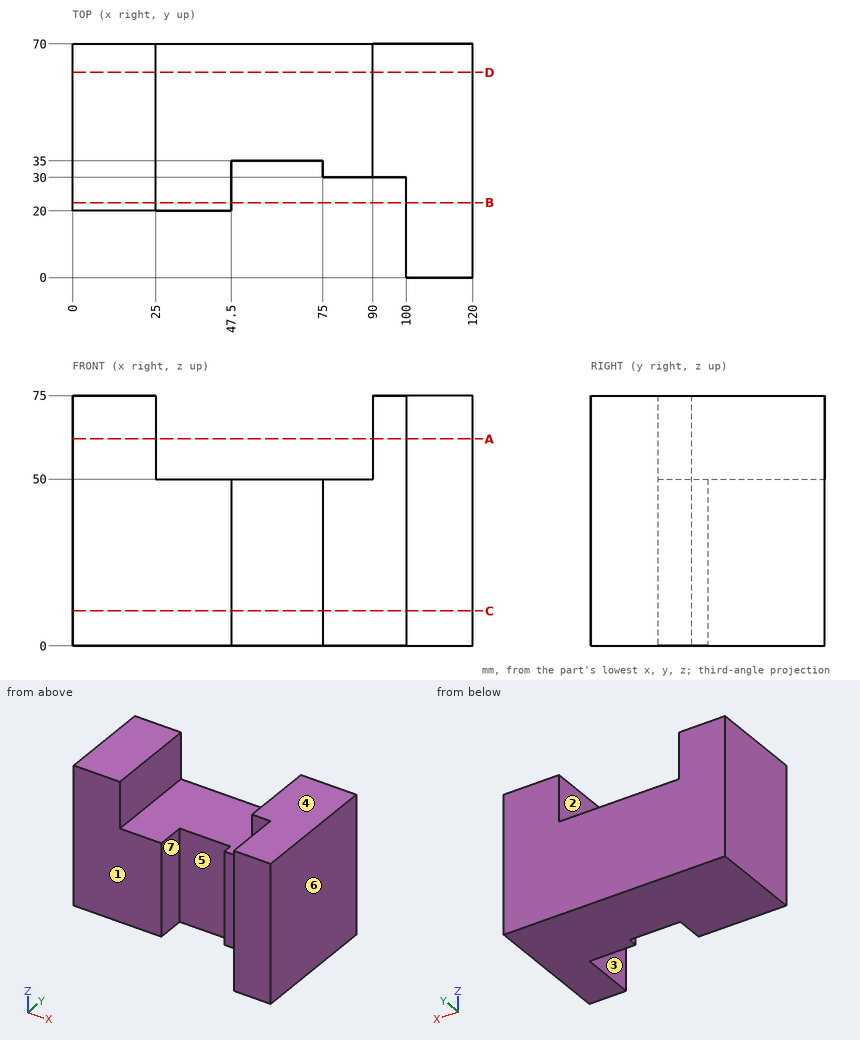
Drawing for the job (mm, zero at the part's lowest x, y, z). A direction names the side the tool comes from. Give positions to 0.01 mm unless a question says otherwise; leave off trailing zeros. Order: outer loops, then holes, each group sorted by start corner. A loop starts at its lowest first (then second) coordinate and runs counter-clockwise, first axis right, second up. Notation, with made-up numbers: (40.25, 8) - (66.25, 8) arc R18 cw to (66.25, 17) - close; hole circle Ø4 at (88.5, 87). An arc over 180 degrees is marked (long way). Use one line per item in the form item = value.
Item 1: Slice it at D-D on y = 61.5. Give the cut face in (x, z).
Solution:
outline = (0, 0) - (120, 0) - (120, 75) - (90, 75) - (90, 50) - (25, 50) - (25, 75) - (0, 75) - close
Item 2: Two-plate mould, pull along X, no slides. Class the marked faces 4, 5, 6 and 7: released by +X, released by -X, zero draft, split by the parting line, or undercut.
Solution:
face_4 = zero draft
face_5 = undercut
face_6 = released by +X
face_7 = undercut
Item 3: Pin check, flat tips, straight feed: pin 1 Ø1 at (x, y) = (52, 54.5) entering from +Z; pin 2 Ø24 at (x, z) = (34.5, 42.5) entering from -Y. Stop position of each tip, or through.
Solution:
pin_1 = 50
pin_2 = 20
Item 4: Slice it at B-B on y = 22.5. Give the cut face in (x, z).
Solution:
outline = (0, 0) - (47.5, 0) - (47.5, 50) - (25, 50) - (25, 75) - (0, 75) - close; (100, 0) - (120, 0) - (120, 75) - (100, 75) - close
Item 5: Slice it at C-C on z = 10.5. Give the cut face in (x, y).
Solution:
outline = (0, 20) - (47.5, 20) - (47.5, 35) - (75, 35) - (75, 30) - (100, 30) - (100, 0) - (120, 0) - (120, 70) - (0, 70) - close
Item 6: Slice it at A-A on z = 62. Give the cut face in (x, y), and give its area (3 significant figures).
Solution:
outline = (0, 20) - (25, 20) - (25, 70) - (0, 70) - close; (90, 30) - (100, 30) - (100, 0) - (120, 0) - (120, 70) - (90, 70) - close
area = 3,050 mm2
Item 7: Probe probe 1 along X at (y, z) = (21, 41.5); probe 2 along X at (y, z) = (32, 12.5); probe 3 along Y at (x, z) = (72, 27.5). List the from-to ranges inside material, lowest first. Write a range as from..to.
Solution:
probe_1 = 0..47.5, 100..120
probe_2 = 0..47.5, 75..120
probe_3 = 35..70
Item 8: Which spindle directions (+Z, -Z, +X, -X, +Y, -Y) get a long thin tool onto all of the face, cutting with end or side? Do the marked faces 1, 2 and 3. Say none if no direction does.
Solution:
face_1 = +Z, -Z, -X, -Y
face_2 = +Z, +Y, -Y
face_3 = +Z, -Z, -Y
